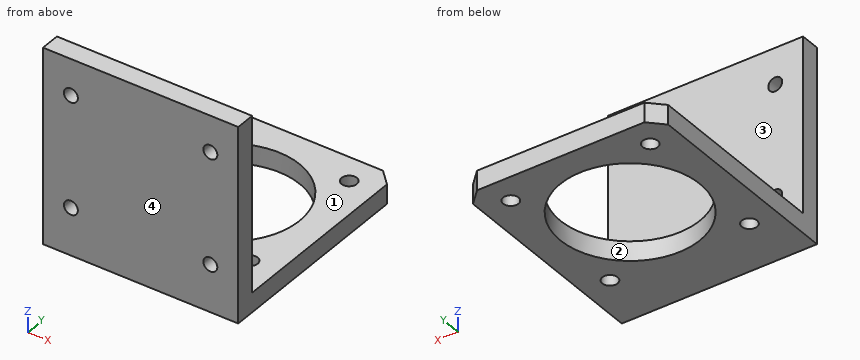
```python
from build123d import *

# Parameters (mm, degrees)
SKETCH1_W           = 70
SKETCH1_H           = 80
SKETCH1_R           = 2.75
SKETCH1_R_2         = 25
BOSS_EXTRUDE1_DEPTH = 7
SKETCH2_W           = 70
SKETCH2_H           = 70
BOSS_EXTRUDE2_DEPTH = 7
SKETCH3_R           = 2.5
CUT_EXTRUDE1_DEPTH  = 7
CHAMFER1_SIZE       = 5


with BuildPart() as part:
    # Sketch1 → Boss-Extrude1 (new body)
    with BuildSketch(Plane.XY):
        Rectangle(SKETCH1_W, SKETCH1_H)
        with Locations((-25, 30)):
            Circle(SKETCH1_R, mode=Mode.SUBTRACT)
        with Locations((25, 30)):
            Circle(SKETCH1_R, mode=Mode.SUBTRACT)
        with Locations((-25, -20)):
            Circle(SKETCH1_R, mode=Mode.SUBTRACT)
        with Locations((25, -20)):
            Circle(SKETCH1_R, mode=Mode.SUBTRACT)
        with Locations((0, 5)):
            Circle(SKETCH1_R_2, mode=Mode.SUBTRACT)
    extrude(amount=BOSS_EXTRUDE1_DEPTH)

    # Sketch2 → Boss-Extrude2 (add)
    with BuildSketch(Plane.XZ.offset(40)):
        with Locations((0, 35)):
            Rectangle(SKETCH2_W, SKETCH2_H)
    extrude(amount=-BOSS_EXTRUDE2_DEPTH)

    # Sketch3 → Cut-Extrude1 (cut)
    with BuildSketch(Plane(origin=(0, -33, 0), x_dir=(1, 0, 0), z_dir=(0, 1, 0))):
        with Locations(Location((-25, -17, 0), (0, 0, 270))):
            Circle(SKETCH3_R)
        with Locations(Location((25, -17, 0), (0, 0, 270))):
            Circle(SKETCH3_R)
        with Locations(Location((-25, -57, 0), (0, 0, 270))):
            Circle(SKETCH3_R)
        with Locations(Location((25, -57, 0), (0, 0, 270))):
            Circle(SKETCH3_R)
    extrude(amount=-CUT_EXTRUDE1_DEPTH, mode=Mode.SUBTRACT)

    # Chamfer1
    chamfer1_edges = [part.edges().sort_by_distance(p)[0] for p in [
        (-35, 40, 3.5),
        (35, 40, 3.5),
    ]]
    chamfer(chamfer1_edges, length=CHAMFER1_SIZE)


solid = part.part
```
The model under review builds one solid part; all positions refer to its coordinate system, in mm. Face numbers are marked on the shaded views. Round coordinates to 2 decimals unless told otherwise and drop trailing zeros. Loops run counter-clockwise (first coordinate to the right, second up) from the corner with the lowest first, then second, coordinate; pieces in that order, holes last.
Item 1: Take a section at B-B (z = 17). Write out the cut boundary in (x, y), then the cut area to 3 significant figures.
Determined:
outline: (-35, -40) - (-27.5, -40) - (-27.5, -33) - (-35, -33) - close; (-22.5, -40) - (22.5, -40) - (22.5, -33) - (-22.5, -33) - close; (27.5, -40) - (35, -40) - (35, -33) - (27.5, -33) - close
area: 420 mm2
Item 2: For line 1 (X direction, y = -37.5, z = 17); line 2 (X direction, y = 31, z = 5.5); line 3 (Z direction, x = 29, y = -14), list the stretches that pass through material, from the lowest coordinate up.
Determined:
line 1: x = -35 to -27.5, -22.5 to 22.5, 27.5 to 35
line 2: x = -35 to -27.56, -22.44 to 22.44, 27.56 to 35
line 3: z = 0 to 7
Item 3: Take a section at C-C (y = 22). Write out the cut boundary in (x, z).
Determined:
outline: (-35, 0) - (-18.33, 0) - (-18.33, 7) - (-35, 7) - close; (18.33, 0) - (35, 0) - (35, 7) - (18.33, 7) - close
Item 4: Clearance check with flat-ended pins moving along their axes: pin 1 Ø5 at (x, z) = (9.5, 17.5) entering from +Y; pin 2 Ø6.5 at (x, z) = (25, 17) entering from -Y; pin 3 Ø6 at (x, y) = (15, -14) entering from +Z. State where each tip first meets the part, or that it passes through.
Determined:
pin 1: stops at y = -33
pin 2: stops at y = -40
pin 3: stops at z = 7
Item 5: Take a section at A-A (x = 1). Write out the cut boundary in (y, z), then the cut area to 3 significant figures.
Determined:
outline: (-40, 0) - (-19.98, 0) - (-19.98, 7) - (-33, 7) - (-33, 70) - (-40, 70) - close; (29.98, 0) - (40, 0) - (40, 7) - (29.98, 7) - close
area: 651 mm2
Item 6: Take a section at D-D (x = -19). Write out the cut boundary in (y, z), then the cut area to 3 significant figures.
Determined:
outline: (-40, 0) - (-11.25, 0) - (-11.25, 7) - (-33, 7) - (-33, 70) - (-40, 70) - close; (21.25, 0) - (40, 0) - (40, 7) - (21.25, 7) - close
area: 774 mm2
Item 7: Mouldability with a two-part tool opening along Y and no side actions: class the marked faces 1, 2, 3 and 4 as released by +Y, released by -Y, zero draft, split by the parting line, or undercut.
Determined:
face 1: zero draft
face 2: undercut
face 3: released by +Y
face 4: released by -Y
